from build123d import *

# Parameters (mm, degrees)
F0_W     = 63.881
F0_H     = 7.874
F1_DEPTH = 3.302
F2_R     = 2.413
F3_DEPTH = 1.778
F5_T     = -1.524
F7_R     = 0.7239
F6_R     = 0.7493
F8_DEPTH = 3.20278


with BuildPart() as f1:
    # F0 (on Top) → F1 (new body)
    with BuildSketch(Plane.XY):
        Rectangle(F0_W, F0_H)
    extrude(amount=F1_DEPTH)

    # F2 (on face) + F0 (on Top) → F3 (join)
    with BuildSketch(Plane.XY.offset(3.302)):
        with BuildLine():
            ThreePointArc((-25.3111, 0), (-27.7241, 2.413), (-30.1371, 0))
            ThreePointArc((-30.1371, 0), (-27.7241, -2.413), (-25.3111, 0))
        make_face()
        with Locations((-19.8501, 0)):
            Circle(F2_R)
        with Locations((-11.9761, 0)):
            Circle(F2_R)
        with Locations((-4.1021, 0)):
            Circle(F2_R)
        with Locations((3.7719, 0)):
            Circle(F2_R)
        with Locations((11.6459, 0)):
            Circle(F2_R)
        with Locations((19.5199, 0)):
            Circle(F2_R)
        with Locations((27.3939, 0)):
            Circle(F2_R)
    with BuildSketch(Plane.XY):
        Rectangle(F0_W, F0_H)
    extrude(amount=F3_DEPTH)

    # F5
    f5_openings = [f1.faces().sort_by_distance(p)[0] for p in [
        (0, 0, 0),
    ]]
    offset(amount=F5_T, openings=f5_openings, kind=Kind.INTERSECTION)

    # F7 (on face) + F6 (on face) → F8 (join)
    with BuildSketch(Plane(origin=(0, 0, 0), x_dir=(1, 0, 0), z_dir=(0, 0, -1))):
        with Locations((-8.001, 0)):
            Circle(F7_R)
        with Locations((-24.003, 0)):
            Circle(F7_R)
        with Locations((-16.002, 0)):
            Circle(F7_R)
    with BuildSketch(Plane(origin=(0, 0, 0), x_dir=(1, 0, 0), z_dir=(0, 0, -1))):
        Circle(F6_R)
        with Locations((7.85095, 0)):
            Circle(F6_R)
        with Locations((15.7019, 0)):
            Circle(F6_R)
        with Locations((23.55285, 0)):
            Circle(F6_R)
    extrude(amount=-F8_DEPTH)


solid = f1.part
Input: part model. Units: mm. Frame: model coordinates. A direction names the side the tool comes from. Coordinates: 2 decimals unless noted, no trailing zeros. Order: outer loops, then holes, each group sorted by start corner. A loop starts at its lowest first (then second) coordinate and runs counter-clockwise, first axis right, second up. Notation, with made-up numbers: M -4.75,-36.5 L 50.25,-36.5 A17 cw 50.25,-30.5 Z; hole C 36.25,-29 d7. An arc over 180 degrees is marked long. Write item = value, one per line. Start each with the question number.
(1) Section D-D on x = 18. Output: boundary loops of the cut face in (y, z).
(2) Section C-C on y = 3. Output: boundary loops of the cut face in (x, z), and give its area (3 significant figures).
(3) Section A-A on z = 0.65. Give the number of separate pieces and of enclosed holes in the cut face, and give its area (3 significant figures).
(4) First-contact query: P1, Ø2, axis at x = -12, y = -0.5, coming from the -Z side; P2, Ø1.4, axis at x = -19.85, y = 0, coming from the -Z side; P3, Ø1, axis at y = -2, z = 4, coming from the -X side. Flat tips, straight axial feed; report the tip coordinate or a pass-through.
(5) Line query: line 1 along Y through (x, z) = (-16, 1.15); line 2 along Y through (x, z) = (29, 1.65); line 3 along Y through (x, z) = (0.5, 1.2). Output: solid intervals per line, ascending. Write a range as [from, to].
(6) Pull-direction query (X, two-part tool) for faces 1 (the cylindrical face through (-26.836, -0.039, 2.655)), 2 (the flat face through (12, 0, 5.08)); classes: released by +X, released by -X, zero draft, split by the parting line, or undercut.
(7) Reachability of faces 3 (the cylindrical face through (6.073, 0.725, 4.179)), 4 (the flat face through (0, 3.937, 2)), 5 (the flat face through (30.416, 0, 1)) from +Z, -Z, +X, -X, +Y, -Y: full face, straight path, thin tool, end or side. Return the list, or none.
(8) Section B-B on x = 0. Output: boundary loops of the cut face in (y, z).
Result set:
q1.outline = M -3.94,0 L -2.41,0 L -2.41,1.78 L 2.41,1.78 L 2.41,0 L 3.94,0 L 3.94,3.3 L 1.87,3.3 L 1.87,5.08 L -1.87,5.08 L -1.87,3.3 L -3.94,3.3 Z
q2.outline = M -31.94,0 L 31.94,0 L 31.94,3.3 L -31.94,3.3 Z
q2.area = 211 mm²
q3.separate_pieces = 8
q3.enclosed_holes = 1
q3.area = 221 mm²
q4.P1 = 1.78
q4.P2 = 3.56
q4.P3 = -29.61
q5.line_1 = [-3.94, -2.41], [-0.72, 0.72], [2.41, 3.94]
q5.line_2 = [-3.94, -2.41], [2.41, 3.94]
q5.line_3 = [-3.94, -2.41], [-0.56, 0.56], [2.41, 3.94]
q6.face_1 = undercut
q6.face_2 = zero draft
q7.face_3 = +Z
q7.face_4 = +Z, -Z, +X, -X, +Y
q7.face_5 = -Z
q8.outline = M -3.94,0 L -2.41,0 L -2.41,1.78 L -0.75,1.78 L -0.75,0 L 0.75,0 L 0.75,1.78 L 2.41,1.78 L 2.41,0 L 3.94,0 L 3.94,3.3 L -3.94,3.3 Z
